from build123d import *

# Parameters (mm, degrees)
ESQUISSE1_W             = 200
ESQUISSE1_H             = 100
BOSS_EXTRU_1_DEPTH      = 20
ESQUISSE2_W             = 25
ESQUISSE2_H             = 25
BOSS_EXTRU_2_DEPTH      = 470
ESQUISSE6_W             = 25
ESQUISSE6_H             = 25
BOSS_EXTRU_3_DEPTH      = 300
ESQUISSE9_R             = 10
ENL_V_MAT_EXTRU_1_DEPTH = 30


with BuildPart() as part:
    # Esquisse1 → Boss.-Extru.1 (new body)
    with BuildSketch(Plane(origin=(0, 0, 0), x_dir=(1, 0, 0), z_dir=(0, 1, 0))):
        Rectangle(ESQUISSE1_W, ESQUISSE1_H)
    extrude(amount=BOSS_EXTRU_1_DEPTH)

    # Esquisse2 → Boss.-Extru.2 (add)
    with BuildSketch(Plane(origin=(0, 0, 0), x_dir=(1, 0, 0), z_dir=(0, 1, 0))):
        Rectangle(ESQUISSE2_W, ESQUISSE2_H)
    extrude(amount=-BOSS_EXTRU_2_DEPTH)

    # Esquisse6 → Boss.-Extru.3 (add)
    with BuildSketch(Plane(origin=(0, 0, -12.5), x_dir=(-1, 0, 0), z_dir=(0, 0, -1))):
        with Locations((0, -457.5)):
            Rectangle(ESQUISSE6_W, ESQUISSE6_H)
    extrude(amount=BOSS_EXTRU_3_DEPTH)

    # Esquisse9 → Enlèv. mat.-Extru.1 (cut)
    with BuildSketch(Plane(origin=(0, -445, 0), x_dir=(1, 0, 0), z_dir=(0, 1, 0))):
        with Locations(Location((0, 296.828421152, 0), (0, 0, 270))):
            Circle(ESQUISSE9_R)
    extrude(amount=-ENL_V_MAT_EXTRU_1_DEPTH, mode=Mode.SUBTRACT)


solid = part.part
The model under review builds one solid part; all positions refer to its coordinate system, in mm. A direction names the side the tool comes from. Round coordinates to 2 decimals unless told otherwise and drop trailing zeros. Loops run counter-clockwise (first coordinate to the right, second up) from the corner with the lowest first, then second, coordinate; pieces in that order, holes last. Notation, with made-up numbers: M 52,3 L 74,3 A32 ccw 74,42 Z; hole C 86,-16.75 d4. An arc over 180 degrees is marked long. Answer as a JSON object with one key per item and string values.
Item 1: Clearance check with flat-ended pins moving along their axes: P1, Ø20, axis at x = 4, y = -160.5, coming from the -Z side; P2, Ø22, axis at x = -47.5, y = 14, coming from the -Z side; P3, Ø4, axis at x = -4.5, z = -86.5, coming from the +Y side. State where each tip first meets the part, or that it passes through.
Check sheet entries:
{"P1": "z = -12.5", "P2": "z = -50", "P3": "y = -445"}
Item 2: We need section C-C, the plane x = 55.5. State the section outline as (y, z) points.
Check sheet entries:
{"outline": "M 0,-50 L 20,-50 L 20,50 L 0,50 Z"}
Item 3: We need section D-D, the plane y = -123.5. State the section outline as (x, z) points, and give its area (3 significant figures).
Check sheet entries:
{"outline": "M -12.5,-12.5 L 12.5,-12.5 L 12.5,12.5 L -12.5,12.5 Z", "area": "625 mm2"}
Item 4: Tool access review of faces 1 (the face through (-12.5, -306, -5)), 2 (the face through (100, 10, 1)), 3 (the face through (0, -445, -160)), 4 (the face through (0, -470, -148)), 5 (the face through (12.5, -306, -5)): name each direction out of +Z, -Z, +X, -X, +Y, -Y from which nothing blocks a thin tool from reaching the whole face with its end or side.
Check sheet entries:
{"face 1": "+Z, -Z, -X, -Y", "face 2": "+Z, -Z, +X, +Y, -Y", "face 3": "-Z, +X, -X", "face 4": "+Z, -Z, +X, -X, -Y", "face 5": "+Z, -Z, +X, -Y"}
Item 5: We need section B-B, the plane z = -2. State the section outline as (x, y) points, and give its area (4 significant figures).
Check sheet entries:
{"outline": "M -100,0 L -12.5,0 L -12.5,-470 L 12.5,-470 L 12.5,0 L 100,0 L 100,20 L -100,20 Z", "area": "15,750 mm2"}
Item 6: We need section A-A, the plane x = 0. State the section outline as (y, z) points, and give its area (4 significant figures).
Check sheet entries:
{"outline": "M -470,-312.5 L -445,-312.5 L -445,-306.83 L -470,-306.83 Z; M -470,-286.83 L -445,-286.83 L -445,-12.5 L 0,-12.5 L 0,-50 L 20,-50 L 20,50 L 0,50 L 0,12.5 L -470,12.5 Z", "area": "20,750 mm2"}
Item 7: For line 1 along X through (y, z) = (-263, 11); line 2 along Y through (x, z) = (-80, 11.5), list the stretches that pass through material, from the lowest coordinate up.
Check sheet entries:
{"line 1": "-12.5 to 12.5", "line 2": "0 to 20"}
Item 8: The part is to be moulded in two halves that separate along Z. For faces 6 (the face through (0, -219, -12.5)), 7 (the face through (0, -232, 12.5)), 8 (the face through (-1, 20, -1)), 9 (the face through (0.44, -457.32, -306.82)), say which applies: +Z half, -Z half, draft (parallel to the pull), parting line (faces both ways), or undercut.
Check sheet entries:
{"face 6": "-Z half", "face 7": "+Z half", "face 8": "draft", "face 9": "undercut"}
